from build123d import *

# Parameters (mm, degrees)
F0_W          = 2032
F0_H          = 203.2
F1_DEPTH      = 25.4
F1_DEPTH_BACK = 25.4
F2_W          = 25.4
F2_H          = 152.4
F3_DEPTH      = 76.2
F4_W          = 25.4
F4_H          = 152.4
F5_DEPTH      = 76.2


with BuildPart() as f1:
    # F0 (on Front) → F1 (new body, two sides)
    with BuildSketch(Plane.XZ) as f1_sk:
        Rectangle(F0_W, F0_H)
    extrude(amount=F1_DEPTH)
    extrude(f1_sk.sketch, amount=-F1_DEPTH_BACK)

    # F2 (on face) → F3 (join)
    with BuildSketch(Plane.YZ.offset(1016)):
        Rectangle(F2_W, F2_H)
    extrude(amount=F3_DEPTH)

    # F4 (on face) → F5 (join)
    with BuildSketch(Plane(origin=(-1016, 0, 0), x_dir=(0, -1, 0), z_dir=(-1, 0, 0))):
        Rectangle(F4_W, F4_H)
    extrude(amount=F5_DEPTH)


solid = f1.part
Input: part model. Units: mm. Frame: model coordinates. A direction names the side the tool comes from. Coordinates: 2 decimals unless noted, no trailing zeros. Loops run counter-clockwise (first coordinate to the right, second up) from the corner with the lowest first, then second, coordinate; pieces in that order, holes last.
Q1. Material intervals for line 1 (X direction, y = -19, z = -35), sorted ascending.
Q2. Set-up query: faces 4 (the face through (1054, -12.7, -1)), 5 (the face through (-14, 25.4, 1)), 6 (the face through (1054, 12.7, -1)). Return all of +Z, -Z, +X, -X, +Y, -Y with unobstructed straight access to the full face (end or side cutting, diameter ignored); none if empty.
Q3. Draft query along Y for faces 1 (the face through (1016, -17, -1)), 2 (the face through (-1054, 12.7, -1)), 3 (the face through (-1054, -12.7, -1)). Return one class per face: +Y half, -Y half, draft (parallel to the pull), parting line (faces both ways), or undercut.
Q4. Cut plane A-A (z = -11.5). Output: boundary loops of the cut face in (x, y), then the cut area to 3 significant figures.
Q5. Contact query for flat-ended pins moving along their axis: pin 1 (23 mm diameter, centred on x = 1065, z = -1.5, fed in from +Y); pin 2 (7.5 mm diameter, centred on x = 1036, y = 5, fed in from -Z); pin 3 (20.5 mm diameter, centred on x = 1041.5, y = 5, fed in from +Z). Output: stop coordinate, or through.
Q6. Cut plane B-B (y = 0). Output: boundary loops of the cut face in (x, z).
Working result:
1. line 1: x = -1016 to 1016
2. face 4: +Z, -Z, +X, -Y
2. face 5: +Z, -Z, +X, -X, +Y
2. face 6: +Z, -Z, +X, +Y
3. face 1: draft
3. face 2: +Y half
3. face 3: -Y half
4. outline: (-1092.2, -12.7) - (-1016, -12.7) - (-1016, -25.4) - (1016, -25.4) - (1016, -12.7) - (1092.2, -12.7) - (1092.2, 12.7) - (1016, 12.7) - (1016, 25.4) - (-1016, 25.4) - (-1016, 12.7) - (-1092.2, 12.7) - close
4. area: 107,000 mm2
5. pin 1: stops at y = 12.7
5. pin 2: stops at z = -76.2
5. pin 3: stops at z = 76.2
6. outline: (-1092.2, -76.2) - (-1016, -76.2) - (-1016, -101.6) - (1016, -101.6) - (1016, -76.2) - (1092.2, -76.2) - (1092.2, 76.2) - (1016, 76.2) - (1016, 101.6) - (-1016, 101.6) - (-1016, 76.2) - (-1092.2, 76.2) - close
